Design review of the part shown in the three views and the two pictorial views. Dimensions are in mm from the part's minimum x, y and z. A direction names the side the tool comes from. Coordinates: 2 decimals unless noted, no trailing zeros. Order: outer loops, then holes, each group sorted by start corner. A loop starts at its lowest first (then second) coordinate and runs counter-clockwise, first axis right, second up. Notation, with made-up numbers: (52, 60.25) -> (99, 60.25) arc R12 cw to (99, 81.25) -> close; hole circle Ø8 at (-14.75, -10.75). An arc over 180 degrees is marked (long way). Answer as a JSON object with one key per item and string values. Group by question number.
1) Wall thickness on L1, parallel to Y at x = 84, z = 7; L2, parallel to Z at x = 48, y = 31; L3, parallel to Z at x = 47, y = 22.5: over which ranges is each line inside the solid? List them lowest first.
2) Add section A-A, the plane y = 3. Write out the cut boundary in (x, z), then the cut area to 3 significant figures.
3) Add section C-C, the plane z = 22.5. Write out the cut boundary in (x, y) (1 decimal).
4) Add section D-D, the plane x = 12. Write out the cut boundary in (y, z).
5) Machinability: for the marked faces 1, 2 and 3, which of the approach directions +Z, -Z, +X, -X, +Y, -Y give a long, thin tool a straight path to every point of the face, cutting with its end or side? Answer none if there is none.
6) For pin 1 (4 mm diameter, centred on x = 37, z = 23, fed in from -Y); pin 2 (10 mm diameter, centred on y = 14.5, z = 16, fed in from -X), all flat-tipped, find the tip position at first contact; note any pin that passes through.
7) Draft analysis for pull direction X (two halves, no side actions). For the marked faces 4, 5 and 6, state which applies: +X half, -X half, draft (parallel to the pull), parting line (faces both ways), or undercut.
8) Add section B-B, the plane y = 12. Write out the cut boundary in (x, z).
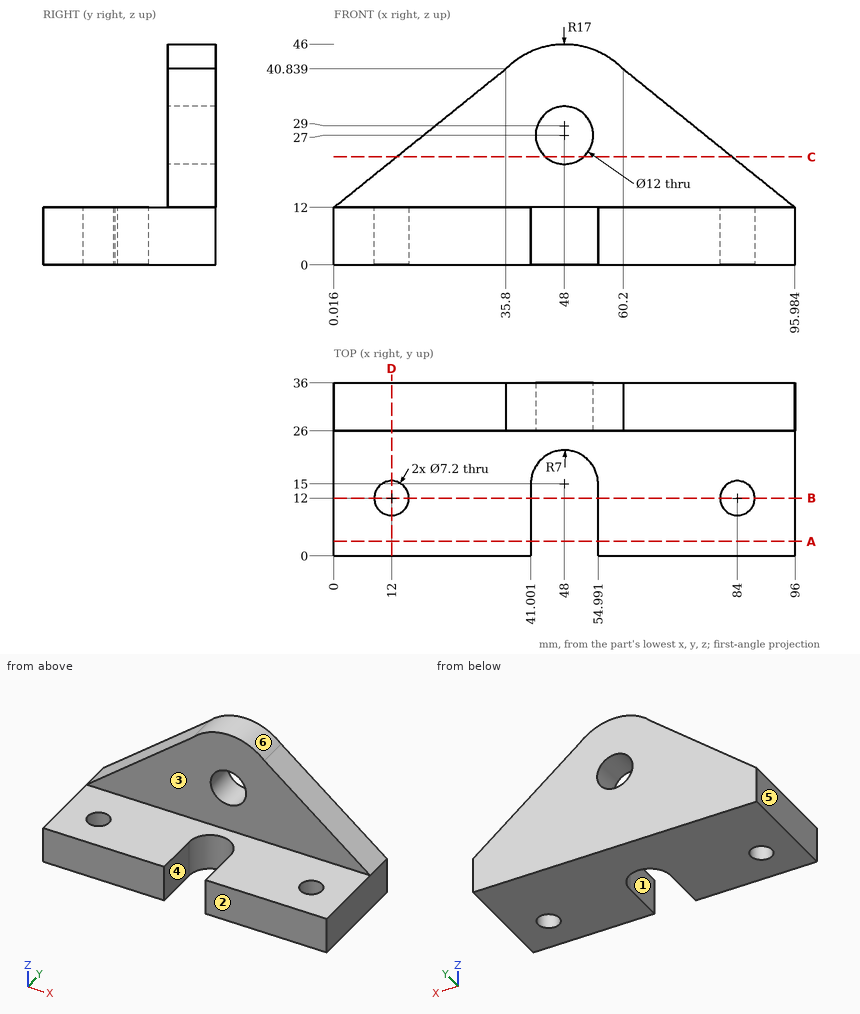
Output values:
{
 "1": {"L1": "y = 0 to 8.4, 15.6 to 36", "L2": "z = 0 to 21, 33 to 46", "L3": "z = 0 to 12"},
 "2": {"outline": "(0, 0) -> (41, 0) -> (41, 12) -> (0, 12) -> close; (54.99, 0) -> (96, 0) -> (96, 12) -> (54.99, 12) -> close", "area": "984 mm²"},
 "3": {"outline": "(13, 26) -> (44, 26) -> (44, 36) -> (13, 36) -> close; (52, 26) -> (83, 26) -> (83, 36) -> (52, 36) -> close"},
 "4": {"outline": "(0, 0) -> (8.4, 0) -> (8.4, 12) -> (0, 12) -> close; (15.6, 0) -> (36, 0) -> (36, 21.66) -> (26, 21.66) -> (26, 12) -> (15.6, 12) -> close"},
 "5": {"face 1": "+Z, -Z, -Y", "face 2": "+Z, -Z, +X, -X, -Y", "face 3": "+Z, +X, -X, -Y"},
 "6": {"pin 1": "stops at y = 26", "pin 2": "stops at x = 0"},
 "7": {"face 4": "undercut", "face 5": "-X half", "face 6": "parting line"},
 "8": {"outline": "(0, 0) -> (8.4, 0) -> (8.4, 12) -> (0, 12) -> close; (15.6, 0) -> (41, 0) -> (41, 12) -> (15.6, 12) -> close; (54.99, 0) -> (80.4, 0) -> (80.4, 12) -> (54.99, 12) -> close; (87.6, 0) -> (96, 0) -> (96, 12) -> (87.6, 12) -> close"}
}
